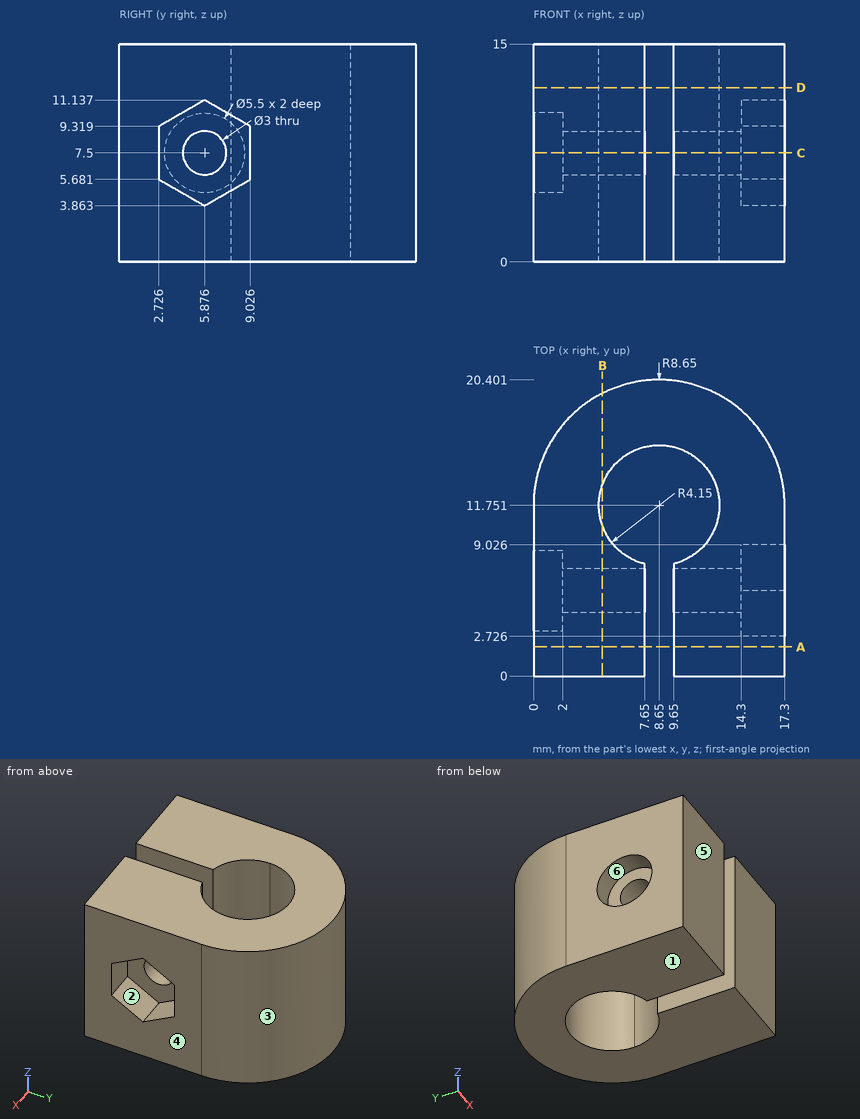
Geometry check sheet. Reference: drawing and pictorial views, mm from the part's lowest x, y, z. A direction names the side the tool comes from. Round coordinates to 2 decimals unless told otherwise and drop trailing zeros. Write each loop counter-clockwise with the first axis right and the second up, starting at its lowest first coordinate (ties: lowest second). Pieces come first, ordered by that corner, then holes.
(1) Mould release check, pull along Y, two halves, no side actions. Record for the marked faces 3, 4, 5 and 6: pulls with the +Y half, pulls with the -Y half, needs draft (parallel to the pull), parting line crosses it, or undercut.
Returned:
face 3: pulls with the +Y half
face 4: needs draft
face 5: pulls with the -Y half
face 6: undercut
(2) Section check D-D (z = 12). Enter the section's corners in (x, y).
Returned:
outline: (0, 0) - (7.65, 0) - (7.65, 7.72) arc R4.15 cw (long way) to (9.65, 7.72) - (9.65, 0) - (17.3, 0) - (17.3, 11.75) arc R8.65 ccw to (0, 11.75) - close
(3) Section check C-C (z = 7.5). Give the number of separate pieces and of enclosed holes in the cut face, plus the area to 3 significant figures.
Returned:
separate pieces: 3
enclosed holes: 0
area: 191 mm2
(4) Depth check by flat-ended pin: pin 1 Ø6 at (y, z) = (15.5, 8.5) entering from -X; pin 2 Ø2 at (x, z) = (10, 2.5) entering from +Y; pin 3 Ø5 at (y, z) = (5.88, 7.5) entering from +X. Enter the tip coordinate at first touch or a pass-through.
Returned:
pin 1: stops at x = 0.03
pin 2: stops at y = 20.39
pin 3: stops at x = 14.3
(5) Material ranges on line 1 (X direction, y = 4.25, z = 12.25); line 2 (X direction, y = 3, z = 7.75); line 3 (Y direction, x = 8.5, z = 1.5), recorded low to high.
Returned:
line 1: x = 0 to 7.65, 9.65 to 17.3
line 2: x = 0 to 7.65, 9.65 to 14.3
line 3: y = 15.9 to 20.4
(6) Access from +Z, -Z, +X, -X, +Y, -Y to the whole of each face (thin tool, end or side, straight path). Record for the marked faces 1 and 2.
Returned:
face 1: -Z, +X, -X, +Y, -Y
face 2: +X
(7) Section check A-A (y = 2). Enter the section's corners in (x, z).
Returned:
outline: (0, 0) - (7.65, 0) - (7.65, 15) - (0, 15) - close; (9.65, 0) - (17.3, 0) - (17.3, 15) - (9.65, 15) - close
(8) Section check B-B (x = 4.75). Enter the section's corners in (y, z) (1 decimal).
Returned:
outline: (0, 0) - (10.3, 0) - (10.3, 15) - (0, 15) - close; (13.2, 0) - (19.5, 0) - (19.5, 15) - (13.2, 15) - close; hole circle Ø3 at (5.9, 7.5)
